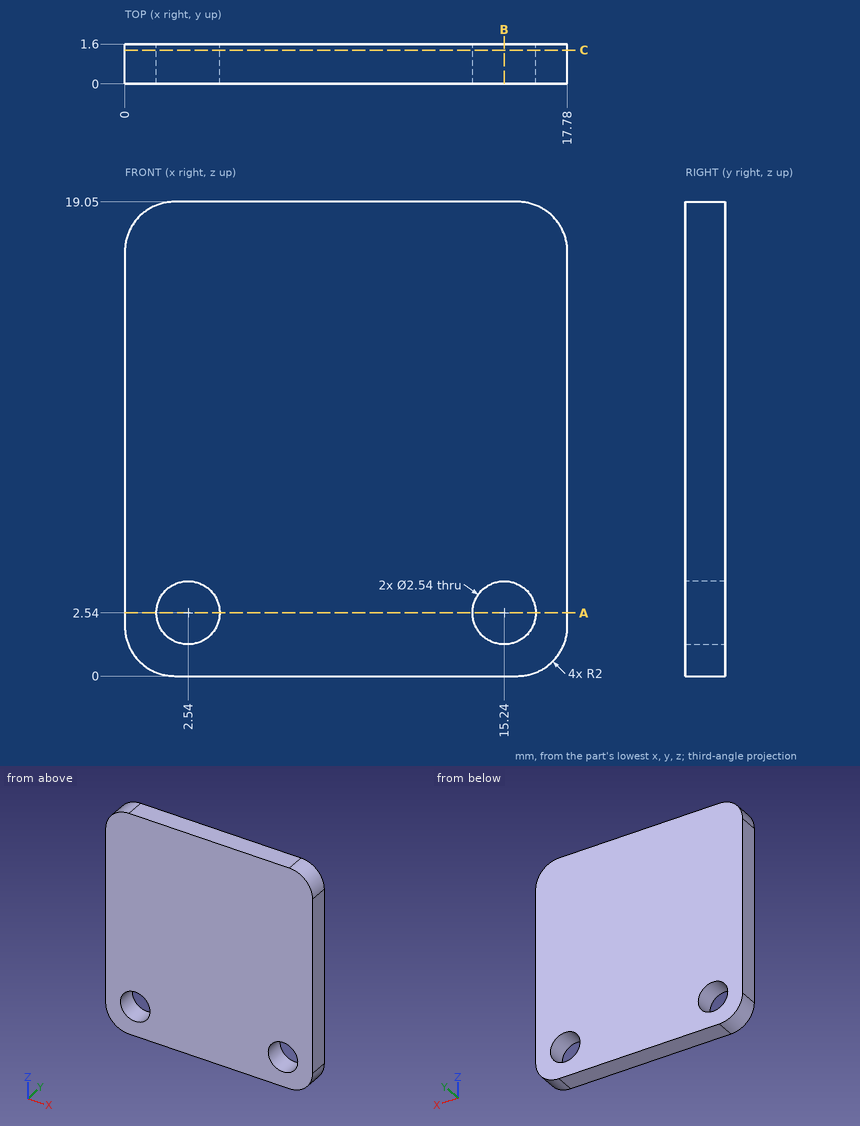
The drawing under review shows one solid part. Ordinate dimensions are in mm from its lowest x, y, z. Coordinates: 2 decimals unless noted, no trailing zeros. Order: outer loops, then holes, each group sorted by start corner. A loop starts at its lowest first (then second) coordinate and runs counter-clockwise, first axis right, second up. Notation, with made-up numbers: (26.25, -29.5) - (54.25, -29.5) arc R18 ccw to (54.25, -2.5) - close; hole circle Ø4 at (57.25, 15). An arc over 180 degrees is marked (long way). Put each result on its own line as item: value.
1) Wall thickness on L1, parallel to X at y = 1.3, z = 2.54; L2, parallel to Z at x = 15.25, y = 0.1; L3, parallel to Z at x = 14.75, y = 0.5: over which ranges is each line inside the solid? List them lowest first. Write a range as from..to.
Response values:
L1: x = 0..1.27, 3.81..13.97, 16.51..17.78
L2: z = 0..1.27, 3.81..19.05
L3: z = 0..1.37, 3.71..19.05
2) Insertion check: P1, Ø2, axis at x = 15.24, z = 2.54, coming from the -Y side. The pin has a flat end and moves straight along its axis. Give the tip position at first contact, or say it passes through.
Response values:
P1: passes through
3) Take a section at A-A, the plane z = 2.54. Give the boundary of the cut face in (x, y), and give its area (3 significant figures).
Response values:
outline: (0, 0) - (1.27, 0) - (1.27, 1.6) - (0, 1.6) - close; (3.81, 0) - (13.97, 0) - (13.97, 1.6) - (3.81, 1.6) - close; (16.51, 0) - (17.78, 0) - (17.78, 1.6) - (16.51, 1.6) - close
area: 20.3 mm²
4) Take a section at C-C, the plane y = 1.35. Give the boundary of the cut face in (x, z).
Response values:
outline: (0, 2) arc R2 ccw to (2, 0) - (15.78, 0) arc R2 ccw to (17.78, 2) - (17.78, 17.05) arc R2 ccw to (15.78, 19.05) - (2, 19.05) arc R2 ccw to (0, 17.05) - close; hole circle Ø2.54 at (2.54, 2.54); hole circle Ø2.54 at (15.24, 2.54)
5) Take a section at B-B, the plane x = 15.24. Give the boundary of the cut face in (y, z), and give its area (3 significant figures).
Response values:
outline: (0, 0) - (1.6, 0) - (1.6, 1.27) - (0, 1.27) - close; (0, 3.81) - (1.6, 3.81) - (1.6, 19.05) - (0, 19.05) - close
area: 26.4 mm²
